Autodesk Inventor part; units mm, degrees
ref_plane "YZ Plane" through (0, 0, 0) normal (1, 0, 0) x (0, 1, 0)
ref_plane "XZ Plane" through (0, 0, 0) normal (0, 1, 0) x (-1, 0, 0)
ref_plane "XY Plane" through (0, 0, 0) normal (0, 0, 1) x (1, 0, 0)
sketch "Skizze1" plane through (0, 0, 0) normal (0, 0, 1) x (1, 0, 0)
  circle A0 centre (0, 0) radius 3.625
  line L0 (0, 47.315) -> (0, -15.615) construction
  line L1 (-9.275, 0) -> (9.275, 0) construction
  circle A1 centre (0, 31.7) radius 3.625
  line L2 (0, 31.7) -> (0, 0) construction
  line L3 (6.625, 31.7) -> (6.625, 0)
  line L4 (-6.625, 0) -> (-6.625, 31.7)
  arc A2 (6.625, 31.7) -> (-6.625, 31.7) centre (0, 31.7) ccw
  arc A3 (-6.625, 0) -> (6.625, 0) centre (0, 0) ccw
  circle A4 centre (0, 31.7) radius 2.625
  circle A5 centre (0, 0) radius 2.625
  point P0 (0, 15.85)
  dimension "d1" = 7.25
  dimension "d2" = 31.7
  dimension "d3" = 1
  dimension "d4" = 3
extrude "Extrusion1" add sketch "Skizze1" along normal blind 3 contours L3 A3 L4 A2
extrude "Extrusion2" add sketch "Skizze1" along normal blind 1 from surface at 3 contours A0 | A1 | L3 A3 L4 A2
properties part number "BeltDriveTestHolder"
Can you work these out from the model? Positions are in its coordinate system, mm. A direction names the side the tool comes from. Give positions to 0.01 mm unless a question says otherwise; leave off trailing zeros. Loops run counter-clockwise (first coordinate to the right, second up) from the corner with the lowest first, then second, coordinate; pieces in that order, holes last. Notation, with made-up numbers: M -1,-1.5 L 8,-1.5 A24 cw 8,21.5 Z; hole C 5,0 d4. An arc over 180 degrees is marked long. Answer in a Markdown table with one row per item.
1. Suppose I cut it at B-B on y = -0.5. Write out the boundary of the cut face in (x, z).
Taken from the geometry:
| item | result |
|---|---|
| outline | M -6.61,0 L -3.59,0 L -3.59,3 L -2.58,3 L -2.58,4 L -6.61,4 Z; M 2.58,3 L 3.59,3 L 3.59,0 L 6.61,0 L 6.61,4 L 2.58,4 Z |
2. Suppose I cut it at D-D on x = 4.75. Write out the boundary of the cut face in (y, z).
Taken from the geometry:
| item | result |
|---|---|
| outline | M -4.62,0 L 36.32,0 L 36.32,4 L -4.62,4 Z |
3. Which directions (+Z, -Z, +X, -X, +Y, -Y) give clear straight access to the entire face, cutting with the end or side of a thin tool? Please do faces 5 (the flat face through (0, 16, 4)), 6 (the flat face through (2, 2, 3)).
Taken from the geometry:
| item | result |
|---|---|
| face 5 | +Z, +X, -X, +Y, -Y |
| face 6 | -Z |
4. Thinking about a two-plate mould opening in X: for faces 1 (the flat face through (6.625, 16, 2)), 2 (the flat face through (0, 16, 0)), 3 (the cylindrical face through (-0.569, 34.263, 3.493)), 4 (the cylindrical face through (-0.146, 38.323, 1.972)), which applies, released by +X, released by -X, zero draft, split by the parting line, or undercut?
Taken from the geometry:
| item | result |
|---|---|
| face 1 | released by +X |
| face 2 | zero draft |
| face 3 | undercut |
| face 4 | split by the parting line |
5. If I drill on line 1 along Y through (x, z) = (0, 1.25) (3 decimals); line 2 along Y through (x, z) = (0, 3.5) (3 decimals); line 3 along Z through (x, y) = (1.5, -3), over which ranges is the centre line in solid material (lowest first)?
Taken from the geometry:
| item | result |
|---|---|
| line 1 | y = -6.625 to -3.625, 3.625 to 28.075, 35.325 to 38.325 |
| line 2 | y = -6.625 to -2.625, 2.625 to 29.075, 34.325 to 38.325 |
| line 3 | z = 3 to 4 |
6. Suppose I cut it at C-C on z = 0.8. Write out the boundary of the cut face in (x, y) (3 decimals).
Taken from the geometry:
| item | result |
|---|---|
| outline | M -6.625,0 A6.625 ccw 6.625,0 L 6.625,31.7 A6.625 ccw -6.625,31.7 Z; hole C 0,0 d7.25; hole C 0,31.7 d7.25 |
7. Suppose I cut it at A-A on x = 0. Write out the boundary of the cut face in (y, z) (3 decimals).
Taken from the geometry:
| item | result |
|---|---|
| outline | M -6.625,0 L -3.625,0 L -3.625,3 L -2.625,3 L -2.625,4 L -6.625,4 Z; M 2.625,3 L 3.625,3 L 3.625,0 L 28.075,0 L 28.075,3 L 29.075,3 L 29.075,4 L 2.625,4 Z; M 34.325,3 L 35.325,3 L 35.325,0 L 38.325,0 L 38.325,4 L 34.325,4 Z |
